Verification items for the finished model (mm, model axes). A direction names the side the tool comes from. Give positions to 0.01 mm unless a question says otherwise; leave off trailing zeros. Write each loop counter-clockwise with the first axis right and the second up, starting at its lowest first coordinate (ties: lowest second). Pieces come first, ordered by that corner, then holes. Notation, with made-up numbers: M 37,-5.75 L 58,-5.75 A19 cw 58,23.25 Z; hole C 68,48.5 d11. An arc over 180 degrees is marked long. Answer as a JSON object with one key per item and string values.
```python
from build123d import *

# Parameters (mm, degrees)
SKETCH_1_W          = 68.077724156
SKETCH_1_H          = 41.280670561
SKETCH_1_W_2        = 62.677724156
SKETCH_1_H_2        = 35.480670561
EXTRUDE_1_DEPTH     = 16
SKETCH_2_W          = 7
SKETCH_2_H          = 13
CUT_EXTRUDE_1_DEPTH = 2.5
SKETCH_3_W          = 16
SKETCH_3_H          = 35.480670561
CUT_EXTRUDE_2_DEPTH = 2.9
SKETCH_4_W          = 68.077724156
SKETCH_4_H          = 41.280670561
EXTRUDE_2_DEPTH     = 3
SKETCH_5_W          = 3
SKETCH_5_H          = 5.5
EXTRUDE_3_DEPTH     = 6.838661
SKETCH_6_W          = 8
SKETCH_6_H          = 15
CUT_EXTRUDE_3_DEPTH = 1
SKETCH_7_W          = 1.5
SKETCH_7_H          = 7
EXTRUDE_4_DEPTH     = 7
SKETCH_8_R          = 1.55
CUT_EXTRUDE_6_DEPTH = 2.5
SKETCH_9_W          = 4
SKETCH_9_H          = 1.5
EXTRUDE_5_DEPTH     = 11
SKETCH_10_W         = 4
SKETCH_10_H         = 1.5
EXTRUDE_6_DEPTH     = 10
CHAMFER_1_SIZE      = 3
FILLET_1_R          = 3
SKETCH_11_W         = 7
SKETCH_11_H         = 1.5
EXTRUDE_7_DEPTH     = 7
SKETCH_12_R         = 1.55
CUT_EXTRUDE_7_DEPTH = 2.5


with BuildPart() as part:
    # 草图1 → 凸台-拉伸1 (new body)
    with BuildSketch(Plane.XY):
        with Locations((-18.003533133, 5.902999581)):
            Rectangle(SKETCH_1_W, SKETCH_1_H)
        with Locations((-18.203533133, 5.902999581)):
            Rectangle(SKETCH_1_W_2, SKETCH_1_H_2, mode=Mode.SUBTRACT)
    extrude(amount=EXTRUDE_1_DEPTH)

    # 草图2 → 切除-拉伸1 (cut)
    with BuildSketch(Plane.ZY.offset(52.042395211)):
        with Locations((3.5, -5.2373357)):
            Rectangle(SKETCH_2_W, SKETCH_2_H)
    extrude(amount=-CUT_EXTRUDE_1_DEPTH, mode=Mode.SUBTRACT)

    # 草图3 → 切除-拉伸2 (cut)
    with BuildSketch(Plane(origin=(16.035328945, 0, 0), x_dir=(0, 0, -1), z_dir=(1, 0, 0))):
        with Locations((-8, 5.902999581)):
            Rectangle(SKETCH_3_W, SKETCH_3_H)
    extrude(amount=-CUT_EXTRUDE_2_DEPTH, mode=Mode.SUBTRACT)

    # 草图4 → 凸台-拉伸2 (add)
    with BuildSketch(Plane.XY.offset(16)):
        with Locations((-18.003533133, 5.902999581)):
            Rectangle(SKETCH_4_W, SKETCH_4_H)
    extrude(amount=EXTRUDE_2_DEPTH)

    # 草图5 → 凸台-拉伸3 (add)
    with BuildSketch(Plane(origin=(16.035328945, 0, 0), x_dir=(0, 0, -1), z_dir=(1, 0, 0))):
        with Locations((-17.5, -6.896027597)):
            Rectangle(SKETCH_5_W, SKETCH_5_H)
        with Locations((-17.5, 19.303972403)):
            Rectangle(SKETCH_5_W, SKETCH_5_H)
    extrude(amount=EXTRUDE_3_DEPTH)

    # 草图6 → 切除-拉伸3 (cut)
    with BuildSketch(Plane.ZY.offset(52.042395211)):
        with Locations((4, -5.2373357)):
            Rectangle(SKETCH_6_W, SKETCH_6_H)
    extrude(amount=-CUT_EXTRUDE_3_DEPTH, mode=Mode.SUBTRACT)

    # 草图7 → 凸台-拉伸4 (add)
    with BuildSketch(Plane.ZY.offset(52.042395211)):
        with Locations((0.75, 15.043334861)):
            Rectangle(SKETCH_7_W, SKETCH_7_H)
    extrude(amount=EXTRUDE_4_DEPTH)

    # 草图8 → 切除-拉伸6 (cut, through all)
    with BuildSketch(Plane.XY.offset(1.5)):
        with Locations((-56.542395211, 15.043334861)):
            Circle(SKETCH_8_R)
    extrude(amount=-CUT_EXTRUDE_6_DEPTH, mode=Mode.SUBTRACT)

    # 草图9 → 凸台-拉伸5 (add)
    with BuildSketch(Plane(origin=(0, 26.543334861, 0), x_dir=(1, 0, 0), z_dir=(0, 1, 0))):
        with Locations((-0.964671055, -18.25)):
            Rectangle(SKETCH_9_W, SKETCH_9_H)
    extrude(amount=EXTRUDE_5_DEPTH)

    # 草图10 → 凸台-拉伸6 (add)
    with BuildSketch(Plane(origin=(0, 0, 17.5), x_dir=(-1, 0, 0), z_dir=(0, 0, -1))):
        with Locations((0.964671055, 36.793334861)):
            Rectangle(SKETCH_10_W, SKETCH_10_H)
    extrude(amount=EXTRUDE_6_DEPTH)

    # 倒角1
    chamfer_1_edges = [part.edges().sort_by_distance(p)[0] for p in [
        (1.035328945, 26.543334861, 18.25),
        (-2.964671055, 26.543334861, 18.25),
    ]]
    chamfer(chamfer_1_edges, length=CHAMFER_1_SIZE)

    # 圆角1
    fillet_1_edges = [part.edges().sort_by_distance(p)[0] for p in [
        (-0.964671055, 36.043334861, 17.5),
    ]]
    fillet(fillet_1_edges, radius=FILLET_1_R)

    # 草图11 → 凸台-拉伸7 (add)
    with BuildSketch(Plane.XZ.offset(14.7373357)):
        with Locations((-17.464671055, 0.75)):
            Rectangle(SKETCH_11_W, SKETCH_11_H)
    extrude(amount=EXTRUDE_7_DEPTH)

    # 草图12 → 切除-拉伸7 (cut, through all)
    with BuildSketch(Plane.XY.offset(1.5)):
        with Locations((-17.464671055, -19.2373357)):
            Circle(SKETCH_12_R)
    extrude(amount=-CUT_EXTRUDE_7_DEPTH, mode=Mode.SUBTRACT)


solid = part.part
```
1) Section check D-D on z = 10.75. Record the boundary of the cut face in (x, y).
Completed:
{"outline": "M -52.04,-14.74 L 16.04,-14.74 L 16.04,-11.84 L -49.54,-11.84 L -49.54,23.64 L 16.04,23.64 L 16.04,26.54 L -52.04,26.54 Z; M -2.96,36.04 L 1.04,36.04 L 1.04,37.54 L -2.96,37.54 Z"}
2) Thickness scan on L1, parallel to Y at x = -0.5, z = 13.75; L2, parallel to Y at x = -24.5, z = 12; L3, parallel to Y at x = -51.5, z = 6.5. Record the ranges inside material, lowest first.
Completed:
{"L1": "y = -14.74 to -11.84, 23.64 to 26.54, 36.04 to 37.54", "L2": "y = -14.74 to -11.84, 23.64 to 26.54", "L3": "y = -14.74 to -12.74, 2.26 to 26.54"}
3) Section check A-A on x = 18. Record the boundary of the cut face in (y, z), and give its area (3 significant figures).
Completed:
{"outline": "M -9.65,16 L -4.15,16 L -4.15,19 L -9.65,19 Z; M 16.55,16 L 22.05,16 L 22.05,19 L 16.55,19 Z", "area": "33.0 mm2"}
4) Section check C-C on y = 0. Record the boundary of the cut face in (x, z), and give its area (3 significant figures).
Completed:
{"outline": "M -52.04,8 L -51.04,8 L -51.04,7 L -49.54,7 L -49.54,16 L 16.04,16 L 16.04,19 L -52.04,19 Z", "area": "226 mm2"}
5) Go/stop test with flat-tipped pins: pin 1 (5.5 mm diameter, centred on x = -12.5, z = 13.5, fed in from +Y); pin 2 (2.5 mm diameter, centred on y = -13, z = 12, fed in from +X); pin 3 (2 mm diameter, centred on y = 20.5, z = 14.5, fed in from +X); pin 4 (2 mm diameter, centred on x = -46, y = 28, fed in from -Z). Record where each tip stops, or that it passes through.
Completed:
{"pin 1": "stops at y = 26.54", "pin 2": "stops at x = 16.04", "pin 3": "stops at x = -49.54", "pin 4": "passes through"}
6) Section check B-B on z = 2.5. Record the boundary of the cut face in (x, y).
Completed:
{"outline": "M -52.04,-14.74 L 16.04,-14.74 L 16.04,-11.84 L -49.54,-11.84 L -49.54,-11.74 L -51.04,-11.74 L -51.04,-12.74 L -52.04,-12.74 Z; M -52.04,2.26 L -51.04,2.26 L -51.04,1.26 L -49.54,1.26 L -49.54,23.64 L 16.04,23.64 L 16.04,26.54 L -52.04,26.54 Z"}
7) Access from +Z, -Z, +X, -X, +Y, -Y to the whole of each face (thin tool, end or side, straight path). Record for faces 5 (the face through (19, -9.646, 18)), 6 (the face through (19, 16.554, 18)), 7 (the face through (-17, -11.837, 8)).
Completed:
{"face 5": "+Z, -Z, +X, -Y", "face 6": "+Z, -Z, +X", "face 7": "-Z, +X"}
8) Release check for a two-part mould opening along Y. For faces 1 (the face through (-51.042, -4.6, 7.2)), 2 (the face through (19, 22.054, 18)), 3 (the face through (-24, 24, 0)), 4 (the face through (-49.542, 10, 8)) record: pulls with the +Y half, pulls with the -Y half, needs draft (parallel to the pull), parting line crosses it, or undercut.
Completed:
{"face 1": "undercut", "face 2": "pulls with the +Y half", "face 3": "needs draft", "face 4": "undercut"}
